Model file for the job. Use its own axes, mm. Face numbers are marked on the shaded views. A direction names the side the tool comes from. Round coordinates to 2 decimals unless told otherwise and drop trailing zeros. Order: outer loops, then holes, each group sorted by start corner. A loop starts at its lowest first (then second) coordinate and runs counter-clockwise, first axis right, second up. Notation, with made-up numbers: (13, 48) - (40, 48) arc R23 cw to (40, 68) - close; hole circle Ø7 at (63, 1). An arc over 180 degrees is marked (long way). Put each result on its own line as item: value. Start each with the question number.
Item 1: Saw through at C-C on x = -8. List the corners of the cut face in (y, z), plus the area to 3 significant figures.
Item 2: Mould opens along Z. For the marked faces 4, 5 and 6 say: pulls with the +Z half, pulls with the -Z half, needs draft (parallel to the pull), parting line crosses it, or undercut.
Item 3: Pin check, flat tips, straight feed: pin 1 Ø2 at (y, z) = (4, 4) entering from +X; pin 2 Ø8 at (x, y) = (-6, -2.5) entering from +Z; pin 3 Ø1.6 at (y, z) = (4.24, 4.24) entering from +X. Stop position of each tip, or through.
Item 4: Saw through at D-D on x = 10. List the corners of the cut face in (y, z), plus the area to 3 significant figures.
Item 5: Probe probe 1 along X at (y, z) = (-4.75, -0.75); probe 2 along X at (y, z) = (-6.5, -1.5); probe 3 along X at (y, z) = (6.75, -4.25). List the from-to ranges inside material, lowest first.
Item 6: Saw through at A-A on x = 13.75. List the corners of the cut face in (y, z), plus the area to 3 significant figures.
Item 7: Which spindle directions (+Z, -Z, +X, -X, +Y, -Y) get a long thin tool onto all of the face, cutting with end or side? Do the marked faces 1, 2 and 3. Say none if no direction does.
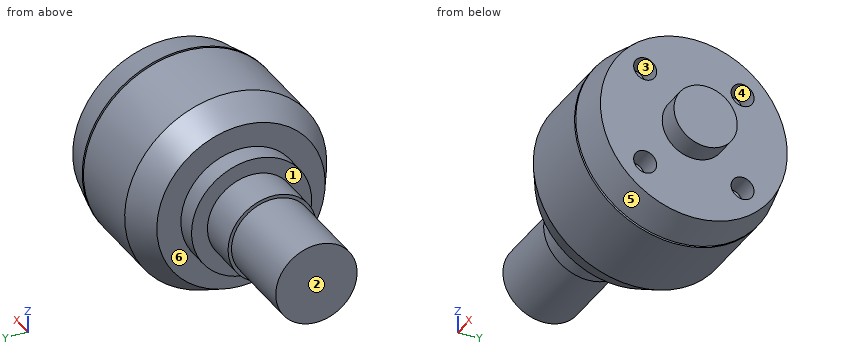
```python
from build123d import *

# Parameters (mm, degrees)
SKETCH3_R          = 1
CUT_EXTRUDE1_DEPTH = 2


with BuildPart() as part:
    # Sketch2 → Revolve1 (revolve)
    with BuildSketch(Plane(origin=(0, 0, 0), x_dir=(1, 0, 0), z_dir=(0, 1, 0))):
        Polygon((-0.295936569, 3.843953818), (-0.295936569, 5.231399235), (1.504063431, 5.231399235), (1.504063431, 7.33120321), (4.097983636, 8.8), (11.097983636, 8.8), (11.097983636, 7.085375335), (11.297983636, 7.085375335), (11.297983636, 8.8), (14.204063431, 8.136308609), (14.204063431, 2.755066744), (16.204063431, 2.755066744), (16.204063431, 0), (-11.295936569, 0), (-11.295936569, 3.544810333), (-3.795936569, 3.544810333), (-3.795936569, 3.843953818), align=None)
    revolve(axis=Axis((16.204063431, 0, 0), (-1, 0, 0)))

    # Sketch3 → Cut-Extrude1 (cut)
    with BuildSketch(Plane(origin=(14.204063431, 0, 0), x_dir=(0, 0, -1), z_dir=(1, 0, 0))):
        with Locations((4.242640687, 4.242640687)):
            Circle(SKETCH3_R)
        with Locations((4.242640687, -4.242640687)):
            Circle(SKETCH3_R)
        with Locations((-4.242640687, -4.242640687)):
            Circle(SKETCH3_R)
        with Locations((-4.242640687, 4.242640687)):
            Circle(SKETCH3_R)
    extrude(amount=-CUT_EXTRUDE1_DEPTH, mode=Mode.SUBTRACT)


solid = part.part
```
Results found:
1. outline: circle Ø7.09 at (0, 0)
1. area: 39.5 mm²
2. face 4: undercut
2. face 5: parting line crosses it
2. face 6: needs draft
3. pin 1: stops at x = 14.2
3. pin 2: stops at z = 3.84
3. pin 3: stops at x = 12.2
4. outline: circle Ø17.6 at (0, 0)
4. area: 243 mm²
5. probe 1: x = -0.3 to 14.2
5. probe 2: x = 1.5 to 14.2
5. probe 3: x = 2.64 to 11.1, 11.3 to 14.2
6. outline: circle Ø16.48 at (0, 0); hole circle Ø2 at (-4.24, -4.24); hole circle Ø2 at (-4.24, 4.24); hole circle Ø2 at (4.24, -4.24); hole circle Ø2 at (4.24, 4.24)
6. area: 201 mm²
7. face 1: -X
7. face 2: +Z, -Z, -X, +Y, -Y
7. face 3: +X
